Autodesk Inventor part; units mm, degrees
ref_plane "Start Plane" through (0, 0, 40) normal (0, 0, 1) x (1, 0, 0)
ref_plane "End Plane" through (0, 0, 380) normal (0, 0, 1) x (1, 0, 0)
ref_plane "YZ Plane" through (0, 0, 0) normal (1, 0, 0) x (0, 1, 0)
ref_plane "Start Plane" through (0, 0, 40) normal (0, 0, 1) x (1, 0, 0)
ref_plane "End Plane" through (0, 0, 380) normal (0, 0, 1) x (1, 0, 0)
sketch "Sketch" plane through (0, 0, 0) normal (0, 0, 1) x (1, 0, 0)
  line L0 (-20, -26) -> (-20, 26)
  line L1 (-16, 30) -> (16, 30)
  line L2 (20, 26) -> (20, -26)
  line L3 (16, -30) -> (-16, -30)
  arc A0 (-20, -26) -> (-16, -30) centre (-16, -26) ccw
  arc A1 (20, 26) -> (16, 30) centre (16, 26) ccw
  arc A2 (-16, 30) -> (-20, 26) centre (-16, 26) ccw
  arc A3 (16, -30) -> (20, -26) centre (16, -26) ccw
  arc A4 (-16, 28) -> (-18, 26) centre (-16, 26) ccw
  line L4 (-16, 28) -> (16, 28)
  arc A5 (18, 26) -> (16, 28) centre (16, 26) ccw
  line L5 (18, 26) -> (18, -26)
  arc A6 (16, -28) -> (18, -26) centre (16, -26) ccw
  line L6 (16, -28) -> (-16, -28)
  arc A7 (-18, -26) -> (-16, -28) centre (-16, -26) ccw
  line L7 (-18, -26) -> (-18, 26)
  line L8 (0, 43.1598) -> (0, -43.1598) construction
  line L9 (-29.1598, 0) -> (29.1598, 0) construction
  dimension "d7" = 4
  dimension "d9" = 40
  dimension "d11" = 60
  dimension "d12" = 2
  dimension "d15" = 20
  dimension "d16" = 30
extrude "Body" add sketch "Sketch" along normal up to surface (340 mm away) from surface at 40
sketch "Sketch3" plane through (0, 0, 0) normal (0, 0, 1) x (1, 0, 0)
  line L0 (0, 0) -> (10, 0)
ref_plane "Work Plane3" through (0, 0, 0) normal (0, -1, 0) x (1, 0, 0)
sketch "Sketch4" plane through (0, 0, 0) normal (0, -1, 0) x (1, 0, 0)
  line L0 (-2, 40) -> (12, 40)
  line L1 (-2, 380) -> (12, 380)
  dimension "d18" = 340
equation "\"d7\" = G_IR"
equation "\"d9\" = G_W"
equation "\"d11\" = G_H"
equation "\"d12\" = G_T"
equation "\"d15\" = 0.5 * d9"
equation "\"d16\" = 0.5 * d11"
equation "\"d3\" = G_L"
equation "\"G_W\" = 40"
equation "\"G_H\" = 60"
equation "\"G_T\" = 2"
equation "\"G_IR\" = 4"
equation "\"G_L\" = d18"
equation "\"G_OFFSET_END\" = 0"
properties part number "ISO 10799-2 - 60x40x2 - 340" material "Steel, Mild"
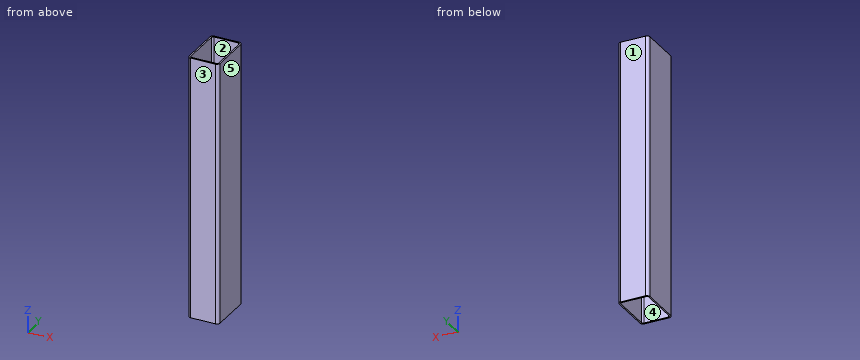
Design review of the part built by this model. Coordinates are the model's own, in mm. Face numbers are marked on the shaded views. A direction names the side the tool comes from. Round coordinates to 2 decimals unless told otherwise and drop trailing zeros. Write each loop counter-clockwise with the first axis right and the second up, starting at its lowest first coordinate (ties: lowest second). Pieces come first, ordered by that corner, then holes.
Item 1: The part is to be moulded in two halves that separate along Y. For the marked faces 1, 2 and 3, say which applies: +Y half, -Y half, draft (parallel to the pull), parting line (faces both ways), or undercut.
Item 2: Clearance check with a flat-ended pin moving along its axis: pin 1 Ø1.5 at (x, y) = (15.5, 13) entering from +Z. State where the tip first meets the part, or that it passes through.
Item 3: We need section C-C on z = 299. Write out the cut boundary in (x, y).
Item 4: We need section A-A on x = -4. Write out the cut boundary in (y, z).
Item 5: For probe 1 along X at (y, z) = (22.5, 122.5); probe 2 along Y at (x, z) = (10.5, 319); probe 3 along X at (y, z) = (-26.5, 64), list the stretches that pass through material, from the lowest coordinate up.
Item 6: We need section B-B on y = 17.5. Write out the cut boundary in (x, z), and give its area (3 significant figures).
Item 7: For the marked faces 4 and 5, list the 3-axis set-ups (+Z, -Z, +X, -X, +Y, -Y) from which the entire face can be reached by the end or side of a thin tool; tool diameter is ignored.
Returned:
1. face 1: +Y half
1. face 2: undercut
1. face 3: -Y half
2. pin 1: passes through
3. outline: (-20, -26) arc R4 ccw to (-16, -30) - (16, -30) arc R4 ccw to (20, -26) - (20, 26) arc R4 ccw to (16, 30) - (-16, 30) arc R4 ccw to (-20, 26) - close; hole (-18, -26) arc R2 ccw to (-16, -28) - (16, -28) arc R2 ccw to (18, -26) - (18, 26) arc R2 ccw to (16, 28) - (-16, 28) arc R2 ccw to (-18, 26) - close
4. outline: (-30, 40) - (-28, 40) - (-28, 380) - (-30, 380) - close; (28, 40) - (30, 40) - (30, 380) - (28, 380) - close
5. probe 1: x = -20 to -18, 18 to 20
5. probe 2: y = -30 to -28, 28 to 30
5. probe 3: x = -19.97 to -17.94, 17.94 to 19.97
6. outline: (-20, 40) - (-18, 40) - (-18, 380) - (-20, 380) - close; (18, 40) - (20, 40) - (20, 380) - (18, 380) - close
6. area: 1,360 mm2
7. face 4: +Z, -Z
7. face 5: +Z, -Z, +X, +Y, -Y
